from build123d import *

# Parameters (mm, degrees)
SKETCH1_R           = 125
BOSS_EXTRUDE1_DEPTH = 6
SKETCH2_R           = 50
CUT_EXTRUDE1_DEPTH  = 6
SKETCH3_R           = 7.5
CUT_EXTRUDE2_DEPTH  = 6
CIRPATTERN1_COUNT   = 8


with BuildPart() as part:
    # Sketch1 → Boss-Extrude1 (new body)
    with BuildSketch(Plane(origin=(0, 0, 0), x_dir=(1, 0, 0), z_dir=(0, 1, 0))):
        with Locations(Location((0, 0, 0), (0, 0, 270))):
            Circle(SKETCH1_R)
    extrude(amount=BOSS_EXTRUDE1_DEPTH)

    # Sketch2 → Cut-Extrude1 (cut)
    with BuildSketch(Plane(origin=(0, 6, 0), x_dir=(1, 0, 0), z_dir=(0, 1, 0))):
        with Locations(Location((0, 0, 0), (0, 0, 270))):
            Circle(SKETCH2_R)
    extrude(amount=-CUT_EXTRUDE1_DEPTH, mode=Mode.SUBTRACT)

    # Sketch3 → Cut-Extrude2 (cut)
    with BuildSketch(Plane(origin=(0, 6, 0), x_dir=(1, 0, 0), z_dir=(0, 1, 0))):
        with Locations(Location((0, 107.5, 0), (0, 0, 270))):
            Circle(SKETCH3_R)
    cut_extrude2 = extrude(amount=-CUT_EXTRUDE2_DEPTH, mode=Mode.SUBTRACT)

    # CirPattern1: Cut-Extrude2 ×8 about axis
    cirpattern1_axis = Axis((0, 0, 0), (0, 1, 0))
    for i in range(1, CIRPATTERN1_COUNT):
        add(cut_extrude2.rotate(cirpattern1_axis, i * 360 / CIRPATTERN1_COUNT), mode=Mode.SUBTRACT)


solid = part.part
Design review of the part built by this model. Coordinates are the model's own, in mm. Coordinates: 2 decimals unless noted, no trailing zeros. Write each loop counter-clockwise with the first axis right and the second up, starting at its lowest first coordinate (ties: lowest second). Pieces come first, ordered by that corner, then holes. Notation, with made-up numbers: (53, 63) -> (68, 63) arc R6 cw to (68, 67) -> close; hole circle Ø8 at (-19.5, 86). An arc over 180 degrees is marked (long way). Write each question's results on one line, items separated by ' | '. Start each with the question number.
(1) The part is to be moulded in two halves that separate along Z. For faces 1 (the face through (2, 0, 54)), 2 (the face through (5.5, 2.96, -124.88)), 3 (the face through (68.69, 3.04, 77.63)), say which applies: pulls with the +Z half, pulls with the -Z half, needs draft (parallel to the pull), parting line crosses it, or undercut.
(2) Clearance check with flat-ended pins moving along their axes: P1, Ø3, axis at y = 2.5, z = -30.5, coming from the +X side; P2, Ø12, axis at x = 76.01, z = 76.01, coming from the -Y side; P3, Ø2, axis at y = 1.5, z = -97, coming from the -X side; P4, Ø2, axis at y = 1, z = -34.5, coming from the +X side. State where each tip first meets the part, or that it passes through.
(3) Take a section at B-B on z = 27.5. Write out the cut boundary in (x, y).
(4) Take a section at C-C on y = 2. Give the number of separate pieces and of enclosed holes in the cut face, and give its area (3 significant figures).
(5) For line 1 along Z through (x, y) = (71, 5.4); line 2 along Z through (x, y) = (81, 2.35); line 3 along X through (y, z) = (2.15, 5), list the stretches that pass through material, from the lowest coordinate up. Write a range as from..to.
(6) Take a section at D-D on x = -107.5. Write out the cut boundary in (y, z).
(7) Take a section at A-A on z = 0. Write out the cut boundary in (x, y).
Results found:
1) face 1: needs draft | face 2: parting line crosses it | face 3: undercut
2) P1: stops at x = 121.59 | P2: passes through | P3: stops at x = -80.06 | P4: stops at x = 120.43
3) outline: (-121.94, 0) -> (-41.76, 0) -> (-41.76, 6) -> (-121.94, 6) -> close; (41.76, 0) -> (121.94, 0) -> (121.94, 6) -> (41.76, 6) -> close
4) separate pieces: 1 | enclosed holes: 9 | area: 39,800 mm2
5) line 1: z = -102.88..-81.59, -70.44..70.44, 81.59..102.88 | line 2: z = -95.21..-81.62, -70.41..70.41, 81.62..95.21 | line 3: x = -124.9..-113.09, -101.91..-49.75, 49.75..101.91, 113.09..124.9
6) outline: (0, -63.79) -> (6, -63.79) -> (6, -7.5) -> (0, -7.5) -> close; (0, 7.5) -> (6, 7.5) -> (6, 63.79) -> (0, 63.79) -> close
7) outline: (-125, 0) -> (-115, 0) -> (-115, 6) -> (-125, 6) -> close; (-100, 0) -> (-50, 0) -> (-50, 6) -> (-100, 6) -> close; (50, 0) -> (100, 0) -> (100, 6) -> (50, 6) -> close; (115, 0) -> (125, 0) -> (125, 6) -> (115, 6) -> close
